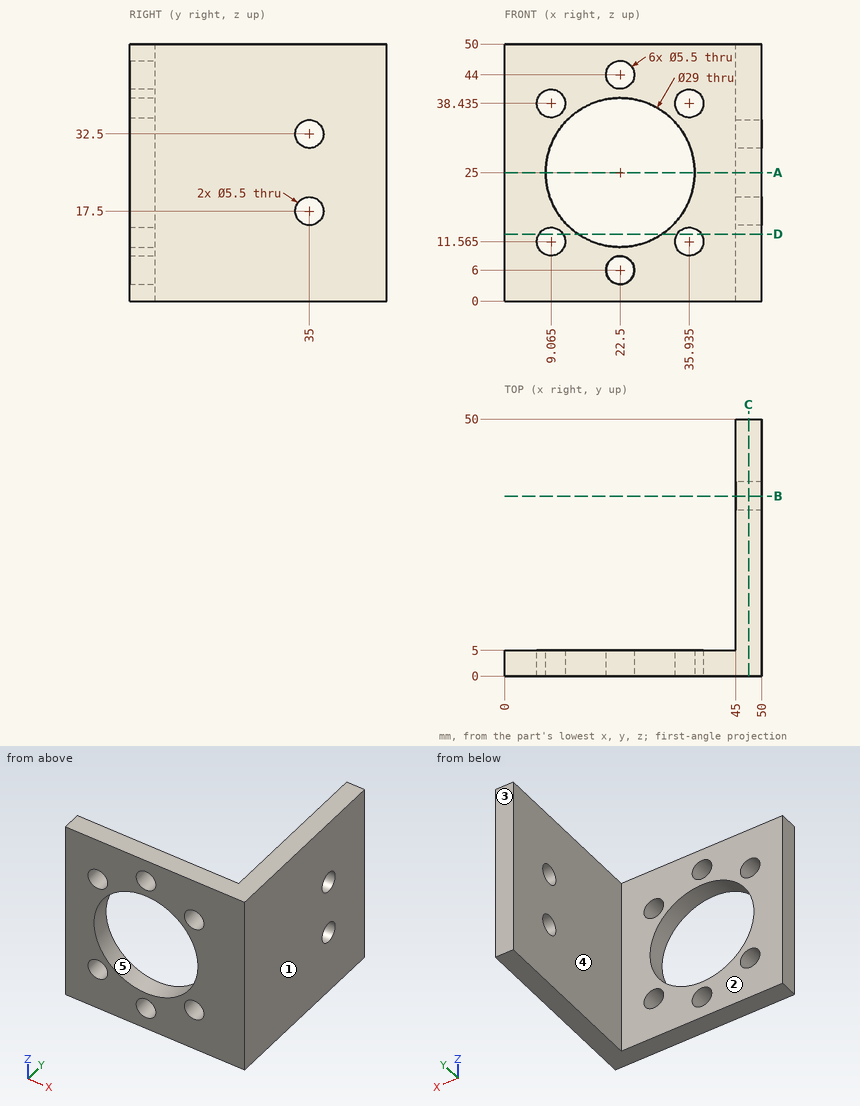
Here's the drawing with two shaded views (mm, measured from the low corner). I have some questions. A direction names the side the tool comes from. Give positions to 0.01 mm unless a question says otherwise; leave off trailing zeros. Write each loop counter-clockwise with the first axis right and the second up, starting at its lowest first coordinate (ties: lowest second). Pieces come first, ordered by that corner, then holes. Notation, with made-up numbers: (75.25, 66.25) -> (130.25, 66.25) arc R5 ccw to (130.25, 71.25) -> close; hole circle Ø9 at (-0.5, -20.75). An arc over 180 degrees is marked (long way). Answer as a JSON object with one key per item and string values. Group by question number.
Item 1: Suppose I cut it at C-C (x = 47.5). Please give me the cut outline in (y, z).
Item 2: For the marked faces 1 and 2, which set-ups out of +Z, -Z, +X, -X, +Y, -Y let a thin tool reach every point of the face, with its end or its side?
Item 3: Please list where these lines run through material, in increasing order: line 1 (Z direction, x = 22.5, y = 1.8); line 2 (X direction, y = 1, z = 6); line 3 (Z direction, x = 10, y = 4.5). Write a range as [from, to].
Item 4: Suppose I cut it at D-D (z = 13). Please give me the cut outline in (x, y).
Item 5: Suppose I cut it at A-A (z = 25). Please give me the cut outline in (x, y), plus the area to 3 significant figures.
Item 6: I'm going to push flat-ended pins straight in: P1, Ø6.5, axis at x = 22.5, z = 44, coming from the +Y side; P2, Ø22.5, axis at y = 23, z = 12.5, coming from the -X side. Where does each tip first touch, or does it pass through?
Item 7: Suppose I cut it at B-B (y = 35). Please give me the cut outline in (x, z).
Item 8: We'd pull the mould along X, two halves only. Please class the marked faces 3, 4 and 5: +X half, -X half, draft (parallel to the pull), parting line (faces both ways), or undercut.
Findings:
{
 "1": {"outline": "(0, 0) -> (50, 0) -> (50, 50) -> (0, 50) -> close; hole circle Ø5.5 at (35, 17.5); hole circle Ø5.5 at (35, 32.5)"},
 "2": {"face 1": "+Z, -Z, +X, +Y, -Y", "face 2": "+Z, -Z, -X, +Y"},
 "3": {"line 1": "z = [0, 3.25], [8.75, 10.5], [39.5, 41.25], [46.75, 50]", "line 2": "x = [0, 19.75], [25.25, 50]", "line 3": "z = [0, 8.98], [14.15, 17.65], [32.35, 35.85], [41.02, 50]"},
 "4": {"outline": "(0, 0) -> (6.72, 0) -> (6.72, 5) -> (0, 5) -> close; (11.41, 0) -> (14.36, 0) -> (14.36, 5) -> (11.41, 5) -> close; (30.64, 0) -> (33.59, 0) -> (33.59, 5) -> (30.64, 5) -> close; (38.28, 0) -> (50, 0) -> (50, 50) -> (45, 50) -> (45, 5) -> (38.28, 5) -> close"},
 "5": {"outline": "(0, 0) -> (8, 0) -> (8, 5) -> (0, 5) -> close; (37, 0) -> (50, 0) -> (50, 50) -> (45, 50) -> (45, 5) -> (37, 5) -> close", "area": "330 mm²"},
 "6": {"P1": "stops at y = 5", "P2": "stops at x = 45"},
 "7": {"outline": "(45, 0) -> (50, 0) -> (50, 14.75) -> (45, 14.75) -> close; (45, 20.25) -> (50, 20.25) -> (50, 29.75) -> (45, 29.75) -> close; (45, 35.25) -> (50, 35.25) -> (50, 50) -> (45, 50) -> close"},
 "8": {"face 3": "draft", "face 4": "-X half", "face 5": "undercut"}
}
